```python
from build123d import *

# Parameters (mm, degrees)
BOSS_EXTRUDE2_DEPTH = 3.175


with BuildPart() as part:
    # Sketch1 → Boss-Extrude2 (new body)
    with BuildSketch(Plane(origin=(0, 0, 0), x_dir=(0, 0, -1), z_dir=(1, 0, 0))):
        Polygon((0, 0), (1.25, 0), (1.25, -3.175), (-21.087781289, -29.796131102), (-17.087781289, -29.796131102), (-6.381931526, -17.037396185), (16.881931526, -17.037396185), (27.587781289, -29.796131102), (31.587781289, -29.796131102), (9.25, -3.175), (9.25, 0), (10.5, 0), (5.25, 4.405273064), align=None)
        Polygon((5.25, -3.175), (14.364632633, -14.037396185), (-3.864632633, -14.037396185), align=None, mode=Mode.SUBTRACT)
    extrude(amount=BOSS_EXTRUDE2_DEPTH)


solid = part.part
```
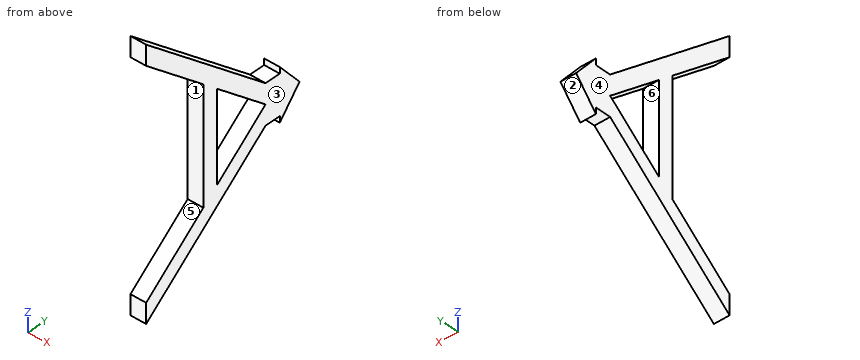
Input: part model. Units: mm. Frame: model coordinates. Face numbers are marked on the shaded views. A direction names the side the tool comes from. Round coordinates to 2 decimals unless told otherwise and drop trailing zeros. Order: outer loops, then holes, each group sorted by start corner. A loop starts at its lowest first (then second) coordinate and runs counter-clockwise, first axis right, second up. Notation, with made-up numbers: (-0.5, 81) - (30.5, 81) arc R33 cw to (30.5, 118) - close; hole circle Ø6 at (-2, 14.5). An arc over 180 degrees is marked (long way). One line per question, with ' | ' between items. Start each with the question number.
1) Contact query for flat-ended pins moving along their axis: P1, Ø0.6, axis at x = 1, z = -0.5, coming from the -Y side; P2, Ø1, axis at x = 1, y = -2, coming from the -Z side; P3, Ø1, axis at x = 1, y = -2, coming from the +Z side. Output: stop coordinate, or through.
2) Pull-direction query (Z, two-part tool) for the marked faces 1, 2 and 3; classes: +Z half, -Z half, draft (parallel to the pull), parting line (faces both ways), or undercut.
3) Cut plane D-D, the plane z = -15. Return the cut outline in (x, y) (3 decimals), then the cut area to 3 significant figures.
4) Ray query, probe 1 along Z at (x, y) = (2.4, -3); probe 2 along Z at (x, y) = (2.05, -19.5); probe 3 along Z at (x, y) = (0.4, -18). Return the intervals inside material, ascending.
5) Cut plane B-B, the plane z = -8. Return the cut outline in (x, y) (3 decimals), then the cut area to 3 significant figures.
6) Cut plane C-C, the plane y = -13. Return the cut outline in (x, z) (3 decimals).
7) Cut plane A-A, the plane x = 0.55. Return the cut outline in (y, z) (3 decimals).
8) Set-up query: the marked faces 4, 5 and 6. Return all of +Z, -Z, +X, -X, +Y, -Y with unobstructed straight access to the full face (end or side cutting, diameter ignored); none if empty.
Worked out:
1) P1: stops at y = -17.04 | P2: stops at z = -9.25 | P3: stops at z = -1.25
2) face 1: undercut | face 2: -Z half | face 3: draft
3) outline: (0, -17.037) - (3.175, -17.037) - (3.175, -10.028) - (0, -10.028) - close | area: 22.3 mm^2
4) probe 1: z = -9.25 to -1.25 | probe 2: z = -22.95 to -18.95, 8.45 to 12.45 | probe 3: z = -21.69 to -17.69, 7.19 to 11.19
5) outline: (0, -17.037) - (3.175, -17.037) - (3.175, -14.037) - (0, -14.037) - close; (0, -6.452) - (3.175, -6.452) - (3.175, 2.098) - (0, 2.098) - close | area: 36.7 mm^2
6) outline: (0, -17.494) - (3.175, -17.494) - (3.175, -13.494) - (0, -13.494) - close; (0, 2.994) - (3.175, 2.994) - (3.175, 6.994) - (0, 6.994) - close
7) outline: (-29.796, -31.588) - (-3.175, -9.25) - (0, -9.25) - (0, -10.5) - (4.405, -5.25) - (0, 0) - (0, -1.25) - (-3.175, -1.25) - (-29.796, 21.088) - (-29.796, 17.088) - (-17.037, 6.382) - (-17.037, -16.882) - (-29.796, -27.588) - close; hole (-14.037, -14.365) - (-3.175, -5.25) - (-14.037, 3.865) - close
8) face 4: +Z, -Z, -X, +Y, -Y | face 5: +X, -X, -Y | face 6: +X, -X
